```python
from build123d import *

# Parameters (mm, degrees)
PAD_DEPTH              = 34.65
SKETCH001_W            = 123.2
SKETCH001_H            = 111.8
POCKET_DEPTH           = 32.65
SKETCH002_W            = 10.2
SKETCH002_H            = 10.2
POCKET001_DEPTH        = 2.4
LINEARPATTERN_COUNT    = 4
LINEARPATTERN_PITCH    = 27.733333
SKETCH003_W            = 10.2
SKETCH003_H            = 10.2
POCKET002_DEPTH        = 2.4
POCKET003_DEPTH        = 2.2
LINEARPATTERN001_COUNT = 2
LINEARPATTERN001_PITCH = 29
SKETCH006_R            = 2.6
POCKET004_DEPTH        = 2.4
LINEARPATTERN002_COUNT = 2
LINEARPATTERN002_PITCH = 33
CHAMFER_SIZE           = 0.5
CHAMFER001_SIZE        = 0.5
CHAMFER002_SIZE        = 0.5
SKETCH013_R            = 0.55
POCKET006_DEPTH        = 2
LINEARPATTERN003_COUNT = 7
LINEARPATTERN003_PITCH = 2.894167
SKETCH014_R            = 0.55
POCKET007_DEPTH        = 2
LINEARPATTERN004_COUNT = 4
LINEARPATTERN004_PITCH = 2.583333
CHAMFER003_SIZE        = 0.2


with BuildPart() as part:
    # Sketch → Pad (new body)
    with BuildSketch(Plane.XY.offset(-7.2)):
        with BuildLine():
            Line((-61.5, -58), (61.2, -58))
            ThreePointArc((61.2, -58), (62.967767, -57.267767), (63.7, -55.5))
            Line((63.7, -55.5), (63.7, 55.5))
            ThreePointArc((63.7, 55.5), (62.967767, 57.267767), (61.2, 58))
            Line((61.2, 58), (-61.5, 58))
            ThreePointArc((-61.5, 58), (-63.267767, 57.267767), (-64, 55.5))
            Line((-64, 55.5), (-64, -55.5))
            ThreePointArc((-64, -55.5), (-63.267767, -57.267767), (-61.5, -58))
        make_face()
    extrude(amount=PAD_DEPTH)

    # Sketch001 → Pocket (cut)
    with BuildSketch(Plane.XY.offset(-7.2)):
        Rectangle(SKETCH001_W, SKETCH001_H)
    extrude(amount=POCKET_DEPTH, mode=Mode.SUBTRACT)

    # Sketch002 (on DatumPlane) → Pocket001 (cut)
    with BuildSketch(Plane(origin=(-64, 0, 0), x_dir=(0, -1, 0), z_dir=(-1, 0, 0))):
        with Locations((-49.08032, 5.1)):
            Rectangle(SKETCH002_W, SKETCH002_H)
    pocket001 = extrude(amount=-POCKET001_DEPTH, mode=Mode.SUBTRACT)

    # LinearPattern: Pocket001 ×4
    with Locations(*[(0, -i * LINEARPATTERN_PITCH, 0) for i in range(1, LINEARPATTERN_COUNT)]):
        add(pocket001, mode=Mode.SUBTRACT)

    # Sketch003 (on DatumPlane) → Pocket002 (cut)
    with BuildSketch(Plane(origin=(-64, 0, 0), x_dir=(0, -1, 0), z_dir=(-1, 0, 0))):
        with Locations((-36.269952, 5.1)):
            Rectangle(SKETCH003_W, SKETCH003_H)
        with Locations((-8.585899, 5.1)):
            Rectangle(SKETCH003_W, SKETCH003_H)
        with Locations((19.356451, 5.1)):
            Rectangle(SKETCH003_W, SKETCH003_H)
        with Locations((47.310611, 5.1)):
            Rectangle(SKETCH003_W, SKETCH003_H)
    extrude(amount=-POCKET002_DEPTH, mode=Mode.SUBTRACT)

    # Sketch004 (on DatumPlane) → Pocket003 (cut)
    with BuildSketch(Plane.YZ.offset(63.7)):
        with BuildLine():
            ThreePointArc((3.703058, 5.203055), (0.111649, 1.611646), (3.703058, -1.979763))
            Line((3.703058, -1.979763), (9.438421, -1.979763))
            ThreePointArc((9.438421, -1.979763), (13.02983, 1.611646), (9.438421, 5.203055))
            Line((3.703058, 5.203055), (9.438421, 5.203055))
        make_face()
    pocket003 = extrude(amount=-POCKET003_DEPTH, mode=Mode.SUBTRACT)

    # LinearPattern001: Pocket003 ×2
    with Locations(*[(0, i * LINEARPATTERN001_PITCH, 0) for i in range(1, LINEARPATTERN001_COUNT)]):
        add(pocket003, mode=Mode.SUBTRACT)

    # Sketch006 (on DatumPlane) → Pocket004 (cut)
    with BuildSketch(Plane.XZ.offset(58)):
        with Locations((56.500076, 4.15)):
            Circle(SKETCH006_R)
    pocket004 = extrude(amount=-POCKET004_DEPTH, mode=Mode.SUBTRACT)

    # LinearPattern002: Pocket004 ×2
    with Locations(*[(-i * LINEARPATTERN002_PITCH, 0, 0) for i in range(1, LINEARPATTERN002_COUNT)]):
        add(pocket004, mode=Mode.SUBTRACT)

    # Chamfer
    chamfer_edges = [part.edges().sort_by_distance(p)[0] for p in [
        (20.900076, -58, 4.15),
        (53.900076, -58, 4.15),
    ]]
    chamfer(chamfer_edges, length=CHAMFER_SIZE)

    # Chamfer001
    chamfer001_edges = [part.edges().sort_by_distance(p)[0] for p in [
        (-64, 55.5, 10.125),
        (-64, 0, -7.2),
        (-64, 0, 27.45),
        (-64, -55.5, 10.125),
        (-64, 54.18032, 5.1),
        (-64, 49.08032, 10.2),
        (-64, 49.08032, 0),
        (-64, 43.98032, 5.1),
        (-64, 41.369952, 5.1),
        (-64, 36.269952, 10.2),
        (-64, 31.169952, 5.1),
        (-64, 36.269952, 0),
        (-64, 26.446987, 5.1),
        (-64, 21.346987, 10.2),
        (-64, 21.346987, 0),
        (-64, 16.246987, 5.1),
        (-64, 13.685899, 5.1),
        (-64, 8.585899, 10.2),
        (-64, 3.485899, 5.1),
        (-64, 8.585899, 0),
        (-64, -1.286347, 5.1),
        (-64, -6.386347, 10.2),
        (-64, -6.386347, 0),
        (-64, -11.486347, 5.1),
        (-64, -14.256451, 5.1),
        (-64, -19.356451, 10.2),
        (-64, -24.456451, 5.1),
        (-64, -19.356451, 0),
        (-64, -29.01968, 5.1),
        (-64, -34.11968, 10.2),
        (-64, -34.11968, 0),
        (-64, -39.21968, 5.1),
        (-64, -42.210611, 5.1),
        (-64, -47.310611, 10.2),
        (-64, -52.410611, 5.1),
        (-64, -47.310611, 0),
    ]]
    chamfer(chamfer001_edges, length=CHAMFER001_SIZE)

    # Chamfer002
    chamfer002_edges = [part.edges().sort_by_distance(p)[0] for p in [
        (63.7, 6.57074, 5.203055),
        (63.7, 35.57074, 5.203055),
    ]]
    chamfer(chamfer002_edges, length=CHAMFER002_SIZE)

    # Sketch013 (on DatumPlane) → Pocket006 (cut)
    with BuildSketch(Plane.XY.offset(27.45)):
        with Locations((55.852455, -36.149361)):
            Circle(SKETCH013_R)
    pocket006 = extrude(amount=-POCKET006_DEPTH, mode=Mode.SUBTRACT)

    # LinearPattern003: Pocket006 ×7
    with Locations(*[(0, i * LINEARPATTERN003_PITCH, 0) for i in range(1, LINEARPATTERN003_COUNT)]):
        add(pocket006, mode=Mode.SUBTRACT)

    # Sketch014 (on DatumPlane) → Pocket007 (cut)
    with BuildSketch(Plane.XY.offset(27.45)):
        with Locations((44.875603, -16.296843)):
            Circle(SKETCH014_R)
    pocket007 = extrude(amount=-POCKET007_DEPTH, mode=Mode.SUBTRACT)

    # LinearPattern004: Pocket007 ×4
    with Locations(*[(0, i * LINEARPATTERN004_PITCH, 0) for i in range(1, LINEARPATTERN004_COUNT)]):
        add(pocket007, mode=Mode.SUBTRACT)

    # Chamfer003
    chamfer003_edges = [part.edges().sort_by_distance(p)[0] for p in [
        (-63.5, 0, 27.45),
        (-62.914214, 56.914214, 27.45),
        (-62.914214, -56.914214, 27.45),
        (-0.15, 57.5, 27.45),
        (-0.15, -57.5, 27.45),
        (62.614214, 56.914214, 27.45),
        (62.614214, -56.914214, 27.45),
        (63.2, 0, 27.45),
        (55.302455, -36.149361, 27.45),
        (55.302455, -33.255194, 27.45),
        (55.302455, -30.361028, 27.45),
        (55.302455, -27.466861, 27.45),
        (55.302455, -24.572694, 27.45),
        (55.302455, -21.678528, 27.45),
        (55.302455, -18.784361, 27.45),
        (44.325603, -16.296843, 27.45),
        (44.325603, -13.71351, 27.45),
        (44.325603, -11.130176, 27.45),
        (44.325603, -8.546843, 27.45),
    ]]
    chamfer(chamfer003_edges, length=CHAMFER003_SIZE)


solid = part.part
```
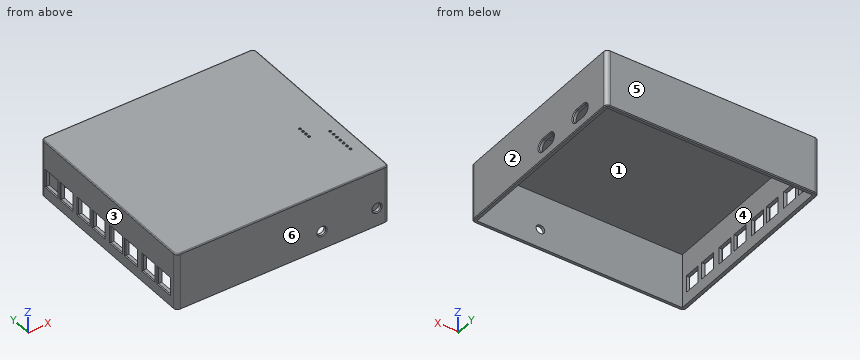
Part model, mm, in its own coordinate system. Face numbers are marked on the shaded views. A direction names the side the tool comes from. Round coordinates to 2 decimals unless told otherwise and drop trailing zeros. Loops run counter-clockwise (first coordinate to the right, second up) from the corner with the lowest first, then second, coordinate; pieces in that order, holes last.
1. Slice it at C-C (x = 7.5). Give the cut face in (y, z), and give its area (3 significant figures).
Solutions:
outline: (-58, -6.7) - (-57.5, -7.2) - (-55.9, -7.2) - (-55.9, 25.45) - (55.9, 25.45) - (55.9, -7.2) - (57.5, -7.2) - (58, -6.7) - (58, 26.95) - (57.64, 27.31) - (57.3, 27.45) - (-57.3, 27.45) - (-57.64, 27.31) - (-58, 26.95) - close
area: 369 mm2
2. Slice it at B-B (z = 23). Give the cut face in (x, y), and give its area (3 significant figures).
Solutions:
outline: (-64, -55.5) arc R2.5 ccw to (-61.5, -58) - (61.2, -58) arc R2.5 ccw to (63.7, -55.5) - (63.7, 55.5) arc R2.5 ccw to (61.2, 58) - (-61.5, 58) arc R2.5 ccw to (-64, 55.5) - close; hole (-61.6, -55.9) - (61.6, -55.9) - (61.6, 55.9) - (-61.6, 55.9) - close
area: 1,030 mm2
3. Flat gauge pins, fed straight in: pin 1 (1.4 mm diameter, centred on x = 44.88, y = -13.71, fed in from -Z); pin 2 (0.9 mm diameter, centred on x = 55.85, y = -36.15, fed in from -Z); pin 3 (8 mm diameter, centred on y = 35, z = 9, fed in from -X); pin 4 (2 mm diameter, centred on x = -63, z = 7, fed in from +Y). Where does each tip first touch, or does it go through?
Solutions:
pin 1: stops at z = 25.45
pin 2: passes through
pin 3: stops at x = -64
pin 4: stops at y = 57.95
4. Slice it at A-A (y = -51). Give the cut face in (x, z), and give its area (3 significant figures).
Solutions:
outline: (-64, -6.7) - (-63.5, -7.2) - (-61.6, -7.2) - (-61.6, 0) - (-63.5, 0) - (-64, -0.5) - close; (-64, 10.7) - (-63.5, 10.2) - (-61.6, 10.2) - (-61.6, 25.45) - (61.6, 25.45) - (61.6, -7.2) - (63.2, -7.2) - (63.7, -6.7) - (63.7, 26.95) - (63.34, 27.31) - (63, 27.45) - (-63.3, 27.45) - (-63.64, 27.31) - (-64, 26.95) - close
area: 377 mm2
5. 3-axis set-ups, long thin cutter, end or side, ignore diameter. For the marked faces 1 and 2: which of +Z, -Z, +X, -X, +Y, -Y reach the whole face in a straight line?
Solutions:
face 1: -Z
face 2: +Z, -Z, +X, +Y, -Y
6. Two-plate mould, pull along Y, no slides. Class the marked faces 3, 4, 5 and 6: pulls with the +Y half, pulls with the -Y half, needs draft (parallel to the pull), parting line crosses it, or undercut.
Solutions:
face 3: needs draft
face 4: undercut
face 5: pulls with the +Y half
face 6: pulls with the -Y half
7. Drill centre lines: line 1 along Y through (x, z) = (-40.5, 18); line 2 along X through (y, z) = (1.5, 24); line 3 along Z through (x, y) = (32, 32.5). Where is each one in solid material? Low to high.
Solutions:
line 1: y = -58 to -55.9, 55.9 to 58
line 2: x = -64 to -61.6, 61.6 to 63.7
line 3: z = 25.45 to 27.45
